```python
from build123d import *

# Parameters (mm, degrees)
SKETCH1_R           = 17.5
SKETCH1_R_2         = 1.5
SKETCH1_R_3         = 4
BOSS_EXTRUDE1_DEPTH = 2
BOSS_EXTRUDE2_DEPTH = 2
SKETCH3_R           = 1.5
BOSS_EXTRUDE4_DEPTH = 2
FILLET1_R           = 1
CHAMFER1_SIZE       = 1
FILLET2_R           = 0.5


with BuildPart() as part:
    # Sketch1 → Boss-Extrude1 (new body)
    with BuildSketch(Plane(origin=(0, 0, 0), x_dir=(1, 0, 0), z_dir=(0, 1, 0))):
        with Locations(Location((0, 0, 0), (0, 0, 270))):
            Circle(SKETCH1_R)
        with Locations(Location((-12.5, 0, 0), (0, 0, 270))):
            Circle(SKETCH1_R_2, mode=Mode.SUBTRACT)
        with Locations(Location((0, -12.5, 0), (0, 0, 270))):
            Circle(SKETCH1_R_2, mode=Mode.SUBTRACT)
        with Locations(Location((12.5, 0, 0), (0, 0, 270))):
            Circle(SKETCH1_R_2, mode=Mode.SUBTRACT)
        with Locations(Location((0, 12.5, 0), (0, 0, 270))):
            Circle(SKETCH1_R_2, mode=Mode.SUBTRACT)
        with Locations(Location((0, 0, 0), (0, 0, 270))):
            Circle(SKETCH1_R_3, mode=Mode.SUBTRACT)
    extrude(amount=BOSS_EXTRUDE1_DEPTH)

    # Sketch2 → Boss-Extrude2 (add)
    with BuildSketch(Plane(origin=(0, 0, 0), x_dir=(1, 0, 0), z_dir=(0, 1, 0))):
        with BuildLine():
            Line((-8, -37.5), (8, -37.5))
            Line((8, -37.5), (8, -15.564382416))
            ThreePointArc((8, -15.564382416), (0, -17.5), (-8, -15.564382416))
            Line((-8, -15.564382416), (-8, -37.5))
        make_face()
    extrude(amount=BOSS_EXTRUDE2_DEPTH)

    # Sketch3 → Boss-Extrude4 (add)
    # profile 1 of 2: a face of its own
    with BuildSketch(Plane(origin=(0, 0, 0), x_dir=(1, 0, 0), z_dir=(0, 1, 0))):
        Polygon((-13.6, -18.5), (-13.6, -22.5), (-8, -24.538233312), (-8, -16.461766688), align=None)
        with Locations(Location((-10.8, -20.5, 0), (0, 0, 270))):
            Circle(SKETCH3_R, mode=Mode.SUBTRACT)
    # profile 2 of 2: a face of its own
    with BuildSketch(Plane(origin=(0, 0, 0), x_dir=(1, 0, 0), z_dir=(0, 1, 0))):
        Polygon((-13.6, -29.5), (-13.6, -33.5), (-8, -35.538233312), (-8, -27.461766688), align=None)
        with Locations(Location((-10.8, -31.5, 0), (0, 0, 270))):
            Circle(SKETCH3_R, mode=Mode.SUBTRACT)
    boss_extrude4 = extrude(amount=BOSS_EXTRUDE4_DEPTH)

    # Mirror1: Boss-Extrude4 across plane
    add(boss_extrude4.mirror(Plane(origin=(0, 0, 0), x_dir=(0, 0, 1), z_dir=(1, 0, 0))))

    # Fillet1
    # the kernel refuses this fillet: 1 mm, written as the material it adds along each edge
    with BuildSketch(Plane(origin=(8, 0, 15.564382416), x_dir=(0.8816627769698464, 0, -0.4718800140987312), z_dir=(0, 1, 0))) as fillet1_piece_1:
        with BuildLine():
            CenterArc((0.59907863, -0.999861528), FILLET1_R, 90.953507264, 60.89009106)
            Line((-0.282584147, -0.527981514), (0, 0))
            ThreePointArc((0, 0), (0.291218778, -0.002423264), (0.582437557, 0))
        make_face()
    extrude(amount=2)
    with BuildSketch(Plane(origin=(-8, 0, 15.564382416), x_dir=(-0.8816627769698451, 0, -0.4718800140987337), z_dir=(0, 1, 0))) as fillet1_piece_2:
        with BuildLine():
            CenterArc((0.59907863, 0.999861528), FILLET1_R, 208.156401676, 60.89009106)
            Line((-0.282584147, 0.527981514), (0, 0))
            ThreePointArc((0, 0), (0.291218778, 0.002423264), (0.582437557, 0))
        make_face()
    extrude(amount=2)
    with BuildSketch(Plane(origin=(-8, 0, 24.538233312), x_dir=(-0.9396926207859061, 0, -0.342020143325675), z_dir=(0, 1, 0)), Plane(origin=(-8, 0, 16.461766688), x_dir=(0, 0, -1), z_dir=(0, 1, 0)), Plane(origin=(-8, 0, 27.461766688), x_dir=(0, 0, -1), z_dir=(0, 1, 0)), Plane(origin=(8, 0, 24.538233312), x_dir=(0, 0, 1), z_dir=(0, 1, 0))) as fillet1_piece_3:
        with BuildLine():
            CenterArc((FILLET1_R * 0.70020753821, FILLET1_R), FILLET1_R, 200, 70)
            Line((-FILLET1_R * 0.239485082576, FILLET1_R * 0.657979856674), (0, 0))
            Line((0, 0), (FILLET1_R * 0.70020753821, 0))
        make_face()
    extrude(amount=2)
    with BuildSketch(Plane(origin=(8, 0, 16.461766688), x_dir=(0, 0, -1), z_dir=(0, 1, 0)), Plane(origin=(8, 0, 27.461766688), x_dir=(0, 0, -1), z_dir=(0, 1, 0))) as fillet1_piece_4:
        with BuildLine():
            CenterArc((FILLET1_R * 0.70020753821, -FILLET1_R), FILLET1_R, 90, 70)
            Line((-FILLET1_R * 0.239485082576, -FILLET1_R * 0.657979856674), (0, 0))
            Line((0, 0), (FILLET1_R * 0.70020753821, 0))
        make_face()
    extrude(amount=2)
    # the kernel refuses this fillet: 1 mm, written as the material it takes off along each edge
    with BuildSketch(Plane(origin=(-13.6, -1.750518846, 22.5), x_dir=(0, 0, -1), z_dir=(0, 1, 0)), Plane(origin=(-13.6, -1.750518846, 18.5), x_dir=(0.9396926207859061, 0, -0.342020143325675), z_dir=(0, 1, 0)), Plane(origin=(-13.6, -1.750518846, 33.5), x_dir=(0, 0, -1), z_dir=(0, 1, 0)), Plane(origin=(-13.6, -1.750518846, 29.5), x_dir=(0.9396926207859078, 0, -0.3420201433256705), z_dir=(0, 1, 0)), Plane(origin=(13.6, -1.750518846, 18.5), x_dir=(0, 0, 1), z_dir=(0, 1, 0)), Plane(origin=(13.6, -1.750518846, 22.5), x_dir=(-0.9396926207859078, 0, 0.3420201433256705), z_dir=(0, 1, 0)), Plane(origin=(13.6, -1.750518846, 29.5), x_dir=(0, 0, 1), z_dir=(0, 1, 0)), Plane(origin=(13.6, -1.750518846, 33.5), x_dir=(-0.9396926207859061, 0, 0.342020143325675), z_dir=(0, 1, 0))) as fillet1_2_piece_1:
        with BuildLine():
            CenterArc((FILLET1_R * 0.70020753821, -FILLET1_R), FILLET1_R, 90, 70)
            Line((-FILLET1_R * 0.239485082576, -FILLET1_R * 0.657979856674), (0, 0))
            Line((0, 0), (FILLET1_R * 0.70020753821, 0))
        make_face()
    extrude(amount=5.501037691, mode=Mode.SUBTRACT)

    # Chamfer1
    chamfer1_edges = [part.edges().sort_by_distance(p)[0] for p in [
        (-8, 1, 37.5),
        (8, 1, 37.5),
    ]]
    chamfer(chamfer1_edges, length=CHAMFER1_SIZE)

    # Fillet2
    fillet2_edges = [part.edges().sort_by_distance(p)[0] for p in [
        (7, 1, 37.5),
        (-7, 1, 37.5),
        (-8, 1, 36.5),
        (8, 1, 36.5),
        (-8, 1, 35.538233312),
        (8, 1, 35.538233312),
    ]]
    fillet(fillet2_edges, radius=FILLET2_R)


solid = part.part
```
Verification items for the finished model (mm, model axes). A direction names the side the tool comes from. Coordinates: 2 decimals unless noted, no trailing zeros. Loops run counter-clockwise (first coordinate to the right, second up) from the corner with the lowest first, then second, coordinate; pieces in that order, holes last. Notation, with made-up numbers: (26.25, 86.25) -> (83.25, 86.25) arc R22 ccw to (83.25, 106.25) -> close; hole circle Ø3 at (16, -5). An arc over 180 degrees is marked (long way). Answer in a Markdown table with one row per item.
1) Section check A-A (z = 0). Record the cut outline in (x, y).
The answers:
| item | result |
|---|---|
| outline | (-17.5, 0) -> (-14, 0) -> (-14, 2) -> (-17.5, 2) -> close; (-11, 0) -> (-4, 0) -> (-4, 2) -> (-11, 2) -> close; (4, 0) -> (11, 0) -> (11, 2) -> (4, 2) -> close; (14, 0) -> (17.5, 0) -> (17.5, 2) -> (14, 2) -> close |
2) Access from +Z, -Z, +X, -X, +Y, -Y to the whole of each face (thin tool, end or side, straight path). Record for faces 1 (the face through (13.6, 1, 20)), 2 (the face through (-13.6, 1, 31)), 3 (the face through (-10.77, 0.99, 17.47)), 4 (the face through (10.77, 0.99, 28.47)).
The answers:
| item | result |
|---|---|
| face 1 | +Z, +X, +Y, -Y |
| face 2 | +Z, -X, +Y, -Y |
| face 3 | -X, +Y, -Y |
| face 4 | +X, +Y, -Y |
3) Section check B-B (x = -10). Record the cut outline in (y, z).
The answers:
| item | result |
|---|---|
| outline | (0, -14.36) -> (2, -14.36) -> (2, 14.36) -> (0, 14.36) -> close; (0, 17.19) -> (2, 17.19) -> (2, 19.23) -> (0, 19.23) -> close; (0, 21.77) -> (2, 21.77) -> (2, 23.81) -> (0, 23.81) -> close; (0, 28.19) -> (2, 28.19) -> (2, 30.23) -> (0, 30.23) -> close; (0, 32.77) -> (2, 32.77) -> (2, 34.81) -> (0, 34.81) -> close |
4) Scan lines: line 1 along X through (y, z) = (1, 31.5); line 2 along Z through (x, y) = (-13, 1.8); line 3 along X through (y, z) = (1.15, 32). Record each from-to range of solid material in increasing order. Write a range as from..to.
The answers:
| item | result |
|---|---|
| line 1 | x = -13.6..-12.3, -9.3..9.3, 12.3..13.6 |
| line 2 | z = -11.72..-1.41, 1.41..11.72, 18.28..22.72, 29.28..33.72 |
| line 3 | x = -13.6..-12.21, -9.39..9.39, 12.21..13.6 |
5) Depth check by flat-ended pin: P1, Ø1.2, axis at y = 1.5, z = 26, coming from the -X side; P2, Ø1, axis at x = -7, y = 1.5, coming from the -Z side. Enter the tip coordinate at first touch or a pass-through.
The answers:
| item | result |
|---|---|
| P1 | stops at x = -8 |
| P2 | stops at z = -16.25 |
6) Draft check along Z on faces 5 (the face through (-3.905, 0.986, -0.867)), 6 (the face through (-10.668, 0.986, 34.567)), 7 (the face through (13.6, 1, 31)). Enter one of: released by +Z, released by -Z, zero draft, split by the parting line, or undercut.
The answers:
| item | result |
|---|---|
| face 5 | undercut |
| face 6 | released by +Z |
| face 7 | zero draft |
7) Section check D-D (y = 1.6). Give the number of separate pieces and of enclosed holes in the cut face, and give its area (3 significant figures).
The answers:
| item | result |
|---|---|
| separate pieces | 1 |
| enclosed holes | 9 |
| area | 1,320 mm2 |
8) Section check C-C (z = 20.5). Record the cut outline in (x, y), and give its area (3 significant figures).
The answers:
| item | result |
|---|---|
| outline | (-13.6, 0) -> (-12.3, 0) -> (-12.3, 2) -> (-13.6, 2) -> close; (-9.3, 0) -> (9.3, 0) -> (9.3, 2) -> (-9.3, 2) -> close; (12.3, 0) -> (13.6, 0) -> (13.6, 2) -> (12.3, 2) -> close |
| area | 42.4 mm2 |
